Input: part model. Units: mm. Frame: model coordinates. Face numbers are marked on the shaded views. A direction names the side the tool comes from. Coordinates: 2 decimals unless noted, no trailing zeros. Loops run counter-clockwise (first coordinate to the right, second up) from the corner with the lowest first, then second, coordinate; pieces in that order, holes last.
Item 1: Section A-A on x = -2.96. Return loops of the section in (y, z).
Item 2: Section D-D on z = 1.75. Return loops of the section in (x, y).
Item 3: Pull-direction query (X, two-part tool) for the marked faces 1, 2 and 3; classes: released by +X, released by -X, zero draft, split by the parting line, or undercut.
Item 4: Section C-C on x = 6.11. Return loops of the section in (y, z), and give its area (3 significant figures).
Item 5: Contact query for a flat-ended pin moving along its axis: P1, Ø2, axis at x = 6.11, z = -1.143, coming from the +Y side. Output: stop coordinate, or through.
Item 6: Reachability of the marked faces 4 and 5 from +Z, -Z, +X, -X, +Y, -Y: full face, straight path, thin tool, end or side. Return the list, or none.
Item 7: Section B-B on y = -3. Return loops of the section in (x, z) (3 decimals), and give its area (3 significant figures).
Item 8: Ray query, line 1 along Y through (x, z) = (3, -2.5); line 2 along Y through (x, z) = (0, -4); line 3 along X through (y, z) = (-4.5, -2.5). Return the intervals inside material, ascending.
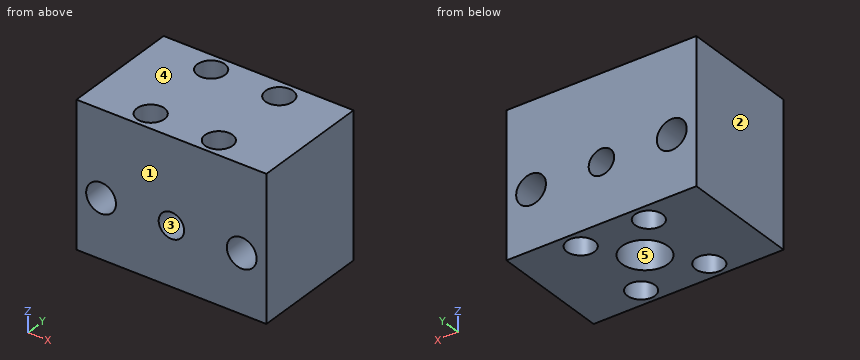
Autodesk Inventor part; units mm, degrees
ref_plane "YZ Plane" through (0, 0, 0) normal (1, 0, 0) x (0, 1, 0)
ref_plane "XZ Plane" through (0, 0, 0) normal (0, 1, 0) x (-1, 0, 0)
ref_plane "XY Plane" through (0, 0, 0) normal (0, 0, 1) x (1, 0, 0)
sketch "Sketch1" plane through (0, 0, 0) normal (0, 0, 1) x (1, 0, 0)
  line L0 (8.25, 5.172) -> (-8.25, 5.172)
  line L1 (-8.25, 5.172) -> (-8.25, -5.172)
  line L2 (-8.25, -5.172) -> (8.25, -5.172)
  line L3 (8.25, -5.172) -> (8.25, 5.172)
  point P0 (0, 0)
  dimension "d19" = 10.344
  dimension "d36" = 16.5
  dimension "d37" = 5.172
extrude "Box" add sketch "Sketch1" along normal mid plane 12.446
sketch "Sketch3" plane through (0, 0, -6.223) normal (0, 0, -1) x (-1, 0, 0)
  line L0 (-5.08, 0) -> (5.08, 0) construction
  line L1 (-4.75, 0) -> (4.75, 0) construction
  circle A0 centre (0, 0) radius 2
  dimension "d35" = 4
extrude "Slot" cut sketch "Sketch3" against normal blind 10.16
sketch "Sketch4" plane through (0, 0, -6.223) normal (0, 0, -1) x (-1, 0, 0)
  circle A0 centre (-2.96, 3.586) radius 1.2
  line L0 (8.25, 5.172) -> (-8.25, 5.172)
  circle A1 centre (0, 0) radius 2
  line L1 (-8.25, 5.172) -> (-8.25, -5.172)
  dimension "d32" = 2.4
  dimension "d34" = 1.586
  dimension "d38" = 3.172
  dimension "d39" = 5.29
extrude "MountingHole" cut sketch "Sketch4" against normal blind 12.5 contours A0
pattern_linear "Mounting Holes" count 2 spacing 5.92 along (-1, 0, 0) count 2 spacing 7.172 along (0, -1, 0) of "MountingHole"
sketch "Sketch6" plane through (-8.25, 5.172, 6.223) normal (0, 1, 0) x (1, 0, 0)
  circle A0 centre (8.25, 7.366) radius 1.105
  point P0 (8.25, 6.223)
  dimension "d20" = 2.21
extrude "CentralSMAHole" cut sketch "Sketch6" against normal blind 12
sketch "Sketch8" plane through (-8.25, 5.172, 6.223) normal (0, 1, 0) x (1, 0, 0)
  circle A0 centre (14.36, 7.366) radius 1.295
  dimension "d23" = 2.59
extrude "SMAMounting" cut sketch "Sketch8" against normal blind 12
pattern_linear "SMAMountingHoles" count 2 spacing 12.22 along (-1, 0, 0) of "SMAMounting"
equation "\"d34\" = 0.5 * d38"
properties part number "NewSinkV2"
Results found:
1. outline: (-5.17, -6.22) - (-4.79, -6.22) - (-4.79, 6.22) - (-5.17, 6.22) - close; (-2.39, -6.22) - (2.39, -6.22) - (2.39, 6.22) - (-2.39, 6.22) - close; (4.79, -6.22) - (5.17, -6.22) - (5.17, 6.22) - (4.79, 6.22) - close
2. outline: (-8.25, -5.17) - (8.25, -5.17) - (8.25, 5.17) - (-8.25, 5.17) - close; hole circle Ø2.4 at (-2.96, -3.59); hole circle Ø2.4 at (-2.96, 3.59); hole circle Ø4 at (0, 0); hole circle Ø2.4 at (2.96, -3.59); hole circle Ø2.4 at (2.96, 3.59)
3. face 1: zero draft
3. face 2: released by -X
3. face 3: undercut
4. outline: (-5.17, -6.22) - (5.17, -6.22) - (5.17, -2.44) - (-5.17, -2.44) - close; (-5.17, 0.15) - (5.17, 0.15) - (5.17, 6.22) - (-5.17, 6.22) - close
4. area: 102 mm2
5. P1: passes through
6. face 4: +Z, +X, -X, +Y, -Y
6. face 5: -Z
7. outline: (-8.25, -6.223) - (-4.007, -6.223) - (-4.007, 6.223) - (-8.25, 6.223) - close; (-1.913, -6.223) - (1.913, -6.223) - (1.913, 6.223) - (-1.913, 6.223) - close; (4.007, -6.223) - (8.25, -6.223) - (8.25, 6.223) - (4.007, 6.223) - close; hole circle Ø2.59 at (-6.11, -1.143); hole circle Ø2.21 at (0, -1.143); hole circle Ø2.59 at (6.11, -1.143)
7. area: 139 mm2
8. line 1: y = -5.17 to -4.79, -2.39 to 2.39, 4.79 to 5.17
8. line 2: y = -5.17 to -2, 2 to 5.17
8. line 3: x = -8.25 to -3.74, -2.18 to 2.18, 3.74 to 8.25
